from build123d import *

# Parameters (mm, degrees)
SKETCH001_R     = 3
POCKET_DEPTH    = 9.001
POCKET001_DEPTH = 5
FILLET_R        = 1
CHAMFER_SIZE    = 0.5


with BuildPart() as part:
    # Sketch → Revolution (revolve)
    with BuildSketch(Plane.XZ):
        Polygon((0, 0), (0, 9), (5.5, 9), (5.5, 5), (7.5, 5), (7.5, 0), align=None)
    revolve(axis=Axis((0, 0, 0), (0, 0, 1)))

    # Sketch001 (on Face1 of Revolution) → Pocket (cut, through all)
    with BuildSketch(Plane(origin=(0, 0, 9), x_dir=(-1, 0, 0), z_dir=(0, 0, 1))):
        Circle(SKETCH001_R)
    extrude(amount=-POCKET_DEPTH, mode=Mode.SUBTRACT)

    # Sketch002 (on Face1 of Pocket) → Pocket001 (cut)
    with BuildSketch(Plane(origin=(0, 0, 9), x_dir=(-1, 0, 0), z_dir=(0, 0, 1))):
        Polygon((4.113621, 2.375), (0, 4.75), (-4.113621, 2.375), (-4.113621, -2.375), (0, -4.75), (4.113621, -2.375), align=None)
    extrude(amount=-POCKET001_DEPTH, mode=Mode.SUBTRACT)

    # Fillet
    fillet_edges = [part.edges().sort_by_distance(p)[0] for p in [
        (-7.5, 0, 5),
    ]]
    fillet(fillet_edges, radius=FILLET_R)

    # Chamfer
    chamfer_edges = [part.edges().sort_by_distance(p)[0] for p in [
        (-5.5, 0, 9),
    ]]
    chamfer(chamfer_edges, length=CHAMFER_SIZE)


solid = part.part
Design review of the part built by this model. Coordinates are the model's own, in mm. A direction names the side the tool comes from. Round coordinates to 2 decimals unless told otherwise and drop trailing zeros. Loops run counter-clockwise (first coordinate to the right, second up) from the corner with the lowest first, then second, coordinate; pieces in that order, holes last. Notation, with made-up numbers: (15, 46.25) -> (36, 46.25) arc R22 ccw to (36, 67.25) -> close; hole circle Ø9 at (-26.5, -2.5). An arc over 180 degrees is marked (long way). Use one line per item in the form item = value. Start each with the question number.
Q1. Machinability: for faces 4 (the face through (1, 3, 4)), 5 (the face through (-0.1, -3.2, 0)), which of the approach directions +Z, -Z, +X, -X, +Y, -Y give a long, thin tool a straight path to every point of the face, cutting with its end or side? Answer none if there is none.
Q2. Draft analysis for pull direction Y (two halves, no side actions). For faces 1 (the face through (5, 3, 5)), 2 (the face through (-7.493, 0.33, 1.972)), 3 (the face through (3, 0, 2)), state which applies: +Y half, -Y half, draft (parallel to the pull), parting line (faces both ways), or undercut.
Q3. We need section B-B on z = 6.5. Give the boundary of the cut face in (x, y) (3 decimals), then the cut area to 3 significant figures.
Q4. We need section A-A on y = 0. Give the boundary of the cut face in (x, z), then the cut area to 3 significant figures.
Q5. We need section C-C on z = 3.25. Give the boundary of the cut face in (x, y), then the cut area to 3 significant figures.
Q6. Wall thickness on line 1 along Y through (x, z) = (0, 2); line 2 along X through (y, z) = (2.5, 1.75); line 3 along X through (y, z) = (2, 7.5): over which ranges is each line inside the solid? List them lowest first. Write a range as [from, to].
Q7. For pin 1 Ø5 at (x, y) = (0, 0) entering from -Z; pin 2 Ø1.5 at (y, z) = (3, 2.5) entering from -X; pin 3 Ø6.5 at (x, y) = (-1, -1.5) entering from +Z; pin 4 Ø2 at (y, z) = (-5, 7.5) entering from +X, all flat-tipped, find the tip position at first contact; note any pin that passes through.
Calculated:
q1.face_4 = +Z
q1.face_5 = -Z, +X, -X, +Y, -Y
q2.face_1 = draft
q2.face_2 = parting line
q2.face_3 = undercut
q3.outline = circle Ø11 at (0, 0); hole (-4.114, -2.375) -> (0, -4.75) -> (4.114, -2.375) -> (4.114, 2.375) -> (0, 4.75) -> (-4.114, 2.375) -> close
q3.area = 36.4 mm²
q4.outline = (-7.5, 0) -> (-3, 0) -> (-3, 4) -> (-4.11, 4) -> (-4.11, 9) -> (-5, 9) -> (-5.5, 8.5) -> (-5.5, 5) -> (-6.5, 5) arc R1 ccw to (-7.5, 4) -> close; (3, 0) -> (7.5, 0) -> (7.5, 4) arc R1 ccw to (6.5, 5) -> (5.5, 5) -> (5.5, 8.5) -> (5, 9) -> (4.11, 9) -> (4.11, 4) -> (3, 4) -> close
q4.area = 53.2 mm²
q5.outline = circle Ø15 at (0, 0); hole circle Ø6 at (0, 0)
q5.area = 148 mm²
q6.line_1 = [-7.5, -3], [3, 7.5]
q6.line_2 = [-7.07, -1.66], [1.66, 7.07]
q6.line_3 = [-5.12, -4.11], [4.11, 5.12]
q7.pin_1 = through
q7.pin_2 = -7.15
q7.pin_3 = 9
q7.pin_4 = 3.77
